Autodesk Inventor part; units mm, degrees
ref_plane "YZ Plane" through (0, 0, 0) normal (1, 0, 0) x (0, 1, 0)
ref_plane "XZ Plane" through (0, 0, 0) normal (0, 1, 0) x (-1, 0, 0)
ref_plane "XY Plane" through (0, 0, 0) normal (0, 0, 1) x (1, 0, 0)
sketch "Эскиз1" plane through (0, 0, 0) normal (0, 1, 0) x (-1, 0, 0)
  line L0 (24, -32.5) -> (-24, -32.5)
  line L1 (-24, -32.5) -> (-24, 32.5)
  line L2 (-24, 32.5) -> (24, 32.5)
  line L3 (24, 32.5) -> (24, -32.5)
  line L4 (24, -32.5) -> (-24, 32.5) construction
  line L5 (-24, -32.5) -> (24, 32.5) construction
  line L6 (-33.6, 0) -> (33.6, 0) construction
  line L7 (0, -45.5) -> (0, 45.5)
  point P0 (0, 0)
  point P1 (0, 0)
  point P2 (0, 0)
  dimension "d0" = 65
  dimension "d1" = 48
extrude "Выдавливание1" add sketch "Эскиз1" along normal mid plane 30
sketch "Эскиз2" plane through (24, -15, -32.5) normal (1, 0, 0) x (0, 0, -1)
  circle A0 centre (-62, 27) radius 1.35
  circle A1 centre (-38, 27) radius 1.35
  circle A2 centre (-38, 3) radius 1.35
  circle A3 centre (-62, 3) radius 1.35
  line L0 (-62, 27) -> (-38, 27) construction
  line L1 (-38, 27) -> (-38, 3) construction
  line L2 (-38, 3) -> (-62, 3) construction
  line L3 (-62, 27) -> (-62, 3) construction
  line L4 (-65, 30) -> (0, 30)
  line L5 (-65, 0) -> (-65, 30)
  point P0 (-32.5, 15)
  dimension "d4" = 2.7
  dimension "d9" = 24
  dimension "d10" = 3
  dimension "d11" = 3
extrude "Выдавливание2" cut sketch "Эскиз2" against normal up to surface (24 mm away)
sketch "Эскиз3" plane through (-24, -15, 32.5) normal (-1, 0, 0) x (0, 0, 1)
  line L0 (-15, 27) -> (-3, 27)
  line L1 (-3, 27) -> (-3, 3)
  line L2 (-3, 3) -> (-15, 3)
  circle A0 centre (-3, 15) radius 1.35
  circle A1 centre (-15, 27) radius 1.35
  circle A2 centre (-15, 3) radius 1.35
  line L3 (-65, 30) -> (0, 30)
  line L4 (0, 30) -> (0, 0)
  point P0 (-32.5, 15)
  dimension "d14" = 24
  dimension "d15" = 12
  dimension "d17" = 2.7
  dimension "d18" = 3
  dimension "d19" = 3
extrude "Выдавливание3" cut sketch "Эскиз3" against normal up to surface (24 mm away)
sketch "Эскиз4" plane through (-24, -15, 32.5) normal (-1, 0, 0) x (0, 0, 1)
  circle A0 centre (-52, 15) radius 3
  line L0 (-78, 15) -> (13, 15)
  line L1 (-65, 0) -> (-65, 30)
  point P0 (-32.5, 15)
  dimension "d22" = 6
  dimension "d23" = 13
extrude "Выдавливание4" add sketch "Эскиз4" along normal blind 7
mirror "Зеркальное отражение1" about plane through (0, 0, 0) normal (1, 0, 0) of "Выдавливание4"
properties part number "рдс150"
Could you check a few things on this model? Use its own coordinates, in mm. A direction names the side the tool comes from. Give positions to 0.01 mm unless a question says otherwise; leave off trailing zeros. Write each loop counter-clockwise with the first axis right and the second up, starting at its lowest first coordinate (ties: lowest second). Pieces come first, ordered by that corner, then holes. Notation, with made-up numbers: (74, -1) -> (120, -1) arc R22 cw to (120, 31) -> close; hole circle Ø3 at (-17, -19). An arc over 180 degrees is marked (long way). Answer as CSV lines item,"result". Start each with the question number.
(1) If we section it at C-C, the plane z = 29.5: Write out the boundary of the cut face in (x, y), and give its area (3 significant figures).
(2) Please list where these lines run through material, in increasing order: line 1 (Y direction, x = 6.25, z = 29.5); line 2 (X direction, y = 12.75, z = -15); line 3 (X direction, y = -11.5, z = 5).
(3) If we section it at D-D, the plane z = -6: Write out the boundary of the cut face in (x, y), and give its area (3 significant figures).
(4) I'm going to push flat-ended pins straight in: pin 1 Ø3.5 at (y, z) = (-12, 29.5) entering from +X; pin 2 Ø4.5 at (y, z) = (12, 29.5) entering from -X; pin 3 Ø2 at (y, z) = (12, 17.5) entering from -X. Where does each tip first touch, or does it pass through?
(5) Which directions (+Z, -Z, +X, -X, +Y, -Y) give clear straight access to the entire face, cutting with the end or side of a thin tool? Please do faces 1 (the face through (31, 0, -19)), 2 (the face through (-12.168, 13.339, 17.324)), 3 (the face through (0, -12, 30)).
(6) If we section it at A-A, the plane z = -19.5: Write out the boundary of the cut face in (x, y), and give its area (3 significant figures).
(7) If we mould it in two halves opening along Z, with no side actions, what happens to faces 4 (the face through (0, -12, 6)), 5 (the face through (-27.5, -0.1, -22.5)), 6 (the face through (0, 0, -32.5))? For each: +Z half, -Z half, draft (parallel to the pull), parting line (faces both ways), or undercut.
(8) If we section it at B-B, the plane y = -12: Write out the boundary of the cut face in (x, z).
Answer list:
1,outline,"(-24, -15) -> (24, -15) -> (24, -13.35) -> (0, -13.35) -> (0, -10.65) -> (24, -10.65) -> (24, 10.65) -> (0, 10.65) -> (0, 13.35) -> (24, 13.35) -> (24, 15) -> (-24, 15) -> (-24, 1.35) -> (0, 1.35) -> (0, -1.35) -> (-24, -1.35) -> close"
1,area,"1,250 mm^2"
2,line 1,"-15 to -13.35, -10.65 to 10.65, 13.35 to 15"
2,line 2,"-24 to 24"
2,line 3,"-24 to 0"
3,outline,"(-24, -15) -> (24, -15) -> (24, 15) -> (-24, 15) -> close"
3,area,"1,440 mm^2"
4,pin 1,"x = 24"
4,pin 2,"x = -24"
4,pin 3,"x = 0"
5,face 1,"+Z, -Z, +X, +Y, -Y"
5,face 2,"-X"
5,face 3,"+X"
6,outline,"(-31, -3) -> (-24, -3) -> (-24, -15) -> (24, -15) -> (24, -3) -> (31, -3) -> (31, 3) -> (24, 3) -> (24, 15) -> (-24, 15) -> (-24, 3) -> (-31, 3) -> close"
6,area,"1,520 mm^2"
7,face 4,"undercut"
7,face 5,"parting line"
7,face 6,"-Z half"
8,outline,"(-24, -32.5) -> (24, -32.5) -> (24, 4.15) -> (0, 4.15) -> (0, 6.85) -> (24, 6.85) -> (24, 28.15) -> (0, 28.15) -> (0, 30.85) -> (24, 30.85) -> (24, 32.5) -> (-24, 32.5) -> (-24, 18.85) -> (0, 18.85) -> (0, 16.15) -> (-24, 16.15) -> close"
